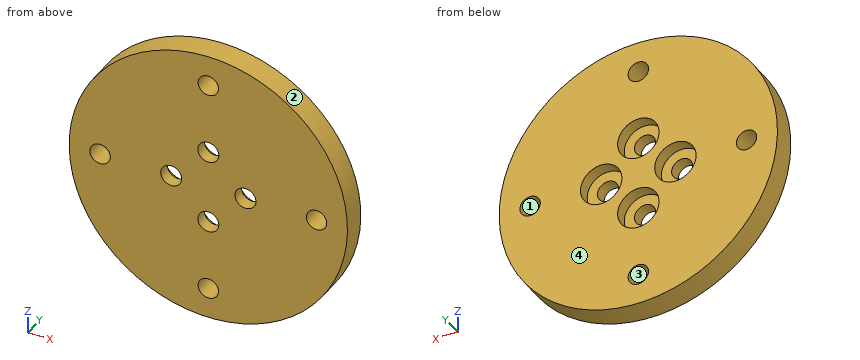
```python
from build123d import *

# Parameters (mm, degrees)
SKETCH_1_R                  = 22.5
EXTRUDE_1_DEPTH             = 4
HOLE_WIZARD_M31_D           = 3.4
HOLE_WIZARD_M31_CBORE_D     = 6.7
HOLE_WIZARD_M31_CBORE_DEPTH = 2
M4X0_71_D                   = 3.3


with BuildPart() as part:
    # Эскиз1 → Бобышка-Вытянуть1 (new body)
    with BuildSketch(Plane(origin=(0, 0, 0), x_dir=(1, 0, 0), z_dir=(0, 1, 0))):
        with Locations(Location((0, 0, 0), (0, 0, 270))):
            Circle(SKETCH_1_R)
    extrude(amount=EXTRUDE_1_DEPTH)

    # Цековка для  винта с полукруглой головкой M31 (through all)
    with Locations(Plane(origin=(0, 4, 0), x_dir=(1, 0, 0), z_dir=(0, 1, 0))):
        with Locations((0, 6), (-6, 0), (0, -6), (6, 0)):
            CounterBoreHole(HOLE_WIZARD_M31_D / 2, HOLE_WIZARD_M31_CBORE_D / 2, HOLE_WIZARD_M31_CBORE_DEPTH)

    # Отверстие обработанное метчиком M4x0.71 (through all)
    with Locations(Plane(origin=(0, 4, 0), x_dir=(1, 0, 0), z_dir=(0, 1, 0))):
        with Locations((-17.5, 0), (0, -17.5), (17.5, 0), (0, 17.5)):
            Hole(M4X0_71_D / 2)


solid = part.part
```
Here's how the part is built. I have some questions about the finished solid (model axes, mm). Face numbers are marked on the shaded views. Coordinates: 2 decimals unless noted, no trailing zeros. Order: outer loops, then holes, each group sorted by start corner. A loop starts at its lowest first (then second) coordinate and runs counter-clockwise, first axis right, second up. Notation, with made-up numbers: M 36.5,87 L 75.5,87 A4 ccw 75.5,91 Z; hole C 79.25,67.5 d9. An arc over 180 degrees is marked long. Answer as a JSON object with one key per item and string values. Group by question number.
(1) Suppose I cut it at A-A, the plane y = 2.75. State how many separate pieces and enclosed holes the cut face has, then the cut area to 3 significant figures.
(2) Suppose I cut it at B-B, the plane x = 0. Please give me the cut outline in (y, z), then the cut area to 3 significant figures.
(3) I need wall thicknesses on probe 1 along Y at (x, z) = (3, 7); probe 2 along Z at (x, y) = (-6, 3.55); probe 3 along X at (y, z) = (0.45, -7). Which ranges of each line are inside material? Lowest first, please.
(4) Suppose I cut it at D-D, the plane x = -18.5. Please give me the cut outline in (y, z), then the cut area to 3 significant figures.
(5) If we mould it in two halves opening along Z, with no side actions, what happens to the marked faces 1, 2, 3 and 4? For each: released by +Z, released by -Z, zero draft, split by the parting line, or undercut.
(6) For pin 1 (3.5 mm diameter, centred on x = 0.5, z = 5.5, fed in from +Y); pin 2 (2 mm diameter, centred on x = 0, z = 6, fed in from -Y); pin 3 (1 mm diameter, centred on y = 2.5, z = 18, fed in from +X); pin 4 (1.5 mm diameter, centred on y = 1, z = 4, fed in from -X), each with a flat end and sliding along its axis, tell me the tip position at first contact or that it passes through.
(7) Suppose I cut it at C-C, the plane z = 6. Please give me the cut outline in (x, y), then the cut area to 3 significant figures.
Values found:
{
 "1": {"separate pieces": "1", "enclosed holes": "8", "area": "1,420 mm^2"},
 "2": {"outline": "M 0,-22.5 L 4,-22.5 L 4,-19.15 L 0,-19.15 Z; M 0,-15.85 L 4,-15.85 L 4,-9.35 L 2,-9.35 L 2,-7.7 L 0,-7.7 Z; M 0,-4.3 L 2,-4.3 L 2,-2.65 L 4,-2.65 L 4,2.65 L 2,2.65 L 2,4.3 L 0,4.3 Z; M 0,7.7 L 2,7.7 L 2,9.35 L 4,9.35 L 4,15.85 L 0,15.85 Z; M 0,19.15 L 4,19.15 L 4,22.5 L 0,22.5 Z", "area": "113 mm^2"},
 "3": {"probe 1": "y = 0 to 2", "probe 2": "z = -21.69 to -3.35, 3.35 to 21.69", "probe 3": "x = -21.38 to -1.37, 1.37 to 21.38"},
 "4": {"outline": "M 0,-12.81 L 4,-12.81 L 4,-1.31 L 0,-1.31 Z; M 0,1.31 L 4,1.31 L 4,12.81 L 0,12.81 Z", "area": "92.0 mm^2"},
 "5": {"face 1": "undercut", "face 2": "split by the parting line", "face 3": "undercut", "face 4": "zero draft"},
 "6": {"pin 1": "stops at y = 2", "pin 2": "passes through", "pin 3": "stops at x = 14.14", "pin 4": "stops at x = -22.26"},
 "7": {"outline": "M -21.69,0 L -1.7,0 L -1.7,2 L -3.35,2 L -3.35,4 L -21.69,4 Z; M 1.7,0 L 21.69,0 L 21.69,4 L 3.35,4 L 3.35,2 L 1.7,2 Z", "area": "153 mm^2"}
}
